```python
from build123d import *

# Parameters (mm, degrees)
EXTRUDE_1_DEPTH = 2


with BuildPart() as part:
    # Model → 凸台-拉伸1 (new body)
    with BuildSketch(Plane.XY):
        Polygon((1022.075950507, 566.466158611), (1022.075950507, 569.466158611), (1024.075950507, 569.466158611), (1024.075950507, 571.466158611), (1028.075950507, 571.466158611), (1028.075950507, 569.466158611), (1032.075950507, 569.466158611), (1032.075950507, 571.466158611), (1036.075950507, 571.466158611), (1036.075950507, 569.466158611), (1038.075950507, 569.466158611), (1038.075950507, 566.466158611), (1040.075950507, 566.466158611), (1040.075950507, 564.466158611), (1038.075950507, 564.466158611), (1038.075950507, 560.466158611), (1040.075950507, 560.466158611), (1040.075950507, 558.466158611), (1038.075950507, 558.466158611), (1038.075950507, 555.466158611), (1036.075950507, 555.466158611), (1036.075950507, 553.466158611), (1032.075950507, 553.466158611), (1032.075950507, 555.466158611), (1028.075950507, 555.466158611), (1028.075950507, 553.466158611), (1024.075950507, 553.466158611), (1024.075950507, 555.466158611), (1022.075950507, 555.466158611), (1022.075950507, 558.466158611), (1020.075950507, 558.466158611), (1020.075950507, 560.466158611), (1022.075950507, 560.466158611), (1022.075950507, 564.466158611), (1020.075950507, 564.466158611), (1020.075950507, 566.466158611), align=None)
    extrude(amount=EXTRUDE_1_DEPTH)


solid = part.part
```
Could you check a few things on this model? Use its own coordinates, in mm. A direction names the side the tool comes from. Coordinates: 2 decimals unless noted, no trailing zeros. Loops run counter-clockwise (first coordinate to the right, second up) from the corner with the lowest first, then second, coordinate; pieces in that order, holes last. Notation, with made-up numbers: M -13.75,30.5 L 0.25,30.5 A18 cw 0.25,52.5 Z; hole C 42.25,10 d1. An arc over 180 degrees is marked long. Put each result on its own line as item: value. Start each with the question number.
(1) Suppose I cut it at A-A on y = 569.75. Please give me the cut outline in (x, z), then the cut area to 3 significant figures.
(2) Suppose I cut it at B-B on x = 1030.5. Please give me the cut outline in (y, z).
(3) Thinking about a two-plate mould opening in Y: for faces 1 (the face through (1039, 566.466, 1)), 2 (the face through (1022.076, 562, 1)), 3 (the face through (1030, 563, 0)), which applies, pulls with the +Y half, pulls with the -Y half, needs draft (parallel to the pull), parting line crosses it, or undercut?
(4) For faces 4 (the face through (1028.076, 554, 1)), 5 (the face through (1028.076, 570, 1)), 6 (the face through (1021, 566.466, 1)), 7 (the face through (1036.076, 554, 1)), which set-ups out of +Z, -Z, +X, -X, +Y, -Y let a thin tool reach every point of the face, with its end or its side?
(5) Will these pins go through, and if not, where does the flat tip stop? P1, Ø0.6, axis at y = 561.5, z = 0.5, coming from the -X side; P2, Ø1, axis at x = 1023.5, z = 0.5, coming from the -Y side; P3, Ø0.6, axis at y = 554.5, z = 1, coming from the +X side.
(6) I need wall thicknesses on line 1 (Y direction, x = 1021.5, z = 1.5); line 2 (X direction, y = 570.75, z = 1.3); line 3 (Y direction, x = 1028.5, z = 0.6). Which ranges of each line are inside material? Lowest first, please. Write a range as from..to.
(7) Suppose I cut it at C-C on y = 562.5. Please give me the cut outline in (x, z).
Solutions:
1. outline: M 1024.08,0 L 1028.08,0 L 1028.08,2 L 1024.08,2 Z; M 1032.08,0 L 1036.08,0 L 1036.08,2 L 1032.08,2 Z
1. area: 16.0 mm2
2. outline: M 555.47,0 L 569.47,0 L 569.47,2 L 555.47,2 Z
3. face 1: pulls with the +Y half
3. face 2: undercut
3. face 3: needs draft
4. face 4: +Z, -Z, -Y
4. face 5: +Z, -Z, +Y
4. face 6: +Z, -Z, -X, +Y
4. face 7: +Z, -Z, +X, -Y
5. P1: stops at x = 1022.08
5. P2: stops at y = 555.47
5. P3: stops at x = 1036.08
6. line 1: y = 558.47..560.47, 564.47..566.47
6. line 2: x = 1024.08..1028.08, 1032.08..1036.08
6. line 3: y = 555.47..569.47
7. outline: M 1022.08,0 L 1038.08,0 L 1038.08,2 L 1022.08,2 Z
